```python
from build123d import *

# Parameters (mm, degrees)
SKETCH1_W           = 42.3
SKETCH1_H           = 42.3
SKETCH1_R           = 11.25
SKETCH1_R_2         = 1.6
BOSS_EXTRUDE1_DEPTH = 4
CHAMFER1_SIZE       = 3


with BuildPart() as part:
    # Sketch1 → Boss-Extrude1 (new body)
    with BuildSketch(Plane.XY):
        Rectangle(SKETCH1_W, SKETCH1_H)
        Circle(SKETCH1_R, mode=Mode.SUBTRACT)
        with Locations((15.717660824, 15.717660824)):
            Circle(SKETCH1_R_2, mode=Mode.SUBTRACT)
        with Locations((-15.279238797, 15.279238797)):
            Circle(SKETCH1_R_2, mode=Mode.SUBTRACT)
        with Locations((-15.279238797, -15.720761203)):
            Circle(SKETCH1_R_2, mode=Mode.SUBTRACT)
        with Locations((15.717660824, -15.282339176)):
            Circle(SKETCH1_R_2, mode=Mode.SUBTRACT)
    extrude(amount=BOSS_EXTRUDE1_DEPTH)

    # Chamfer1
    chamfer1_edges = [part.edges().sort_by_distance(p)[0] for p in [
        (21.15, -21.15, 2),
        (-21.15, -21.15, 2),
        (-21.15, 21.15, 2),
        (21.15, 21.15, 2),
    ]]
    chamfer(chamfer1_edges, length=CHAMFER1_SIZE)


solid = part.part
```
Input: part model. Units: mm. Frame: model coordinates. Coordinates: 2 decimals unless noted, no trailing zeros. Order: outer loops, then holes, each group sorted by start corner. A loop starts at its lowest first (then second) coordinate and runs counter-clockwise, first axis right, second up. Notation, with made-up numbers: (53, -21) - (83, -21) arc R11 cw to (83, -15) - close; hole circle Ø2 at (52, -20.75). An arc over 180 degrees is marked (long way). Put each result on its own line as item: value.
1. Cut plane A-A on y = 0. Return the cut outline in (x, z).
Report:
outline: (-21.15, 0) - (-11.25, 0) - (-11.25, 4) - (-21.15, 4) - close; (11.25, 0) - (21.15, 0) - (21.15, 4) - (11.25, 4) - close
2. Cut plane C-C on z = 1.1. Return the cut outline in (x, y), then the cut area to 3 significant figures.
Report:
outline: (-21.15, -18.15) - (-18.15, -21.15) - (18.15, -21.15) - (21.15, -18.15) - (21.15, 18.15) - (18.15, 21.15) - (-18.15, 21.15) - (-21.15, 18.15) - close; hole circle Ø3.2 at (-15.28, -15.72); hole circle Ø3.2 at (-15.28, 15.28); hole circle Ø22.5 at (0, 0); hole circle Ø3.2 at (15.72, -15.28); hole circle Ø3.2 at (15.72, 15.72)
area: 1,340 mm2
3. Draft query along X for faces 1 (the face through (14.45, -16.26, 1.97)), 2 (the face through (9, -9, 0)), 3 (the face through (-16.878, -15.65, 1.972)), 4 (the face through (-21.15, 0, 2)). Return one class per face: pulls with the +X half, pulls with the -X half, needs draft (parallel to the pull), parting line crosses it, or undercut.
Report:
face 1: undercut
face 2: needs draft
face 3: undercut
face 4: pulls with the -X half
4. Contact query for flat-ended pins moving along their axis: pin 1 Ø3 at (x, y) = (15.72, -15.28) entering from -Z; pin 2 Ø5 at (x, y) = (-15.28, 15.28) entering from +Z. Output: stop coordinate, or through.
Report:
pin 1: passes through
pin 2: stops at z = 4
5. Cut plane B-B on x = 2. Return the cut outline in (y, z).
Report:
outline: (-21.15, 0) - (-11.07, 0) - (-11.07, 4) - (-21.15, 4) - close; (11.07, 0) - (21.15, 0) - (21.15, 4) - (11.07, 4) - close
6. Line query: line 1 along X through (y, z) = (15.5, 0.4); line 2 along Y through (x, z) = (0, 2.9); line 3 along X through (y, z) = (8, 0.55). Output: solid intervals per line, ascending.
Report:
line 1: x = -21.15 to -16.86, -13.69 to 14.13, 17.3 to 21.15
line 2: y = -21.15 to -11.25, 11.25 to 21.15
line 3: x = -21.15 to -7.91, 7.91 to 21.15
